from build123d import *

# Parameters (mm, degrees)
F1_DEPTH = 3
F4_R     = 0.5
F6_R     = 0.1
F7_R     = 3
F8_DEPTH = 25
F9_R     = 0.5
F10_R    = 0.2


with BuildPart() as f1:
    # F0 (on Front) → F1 (new body)
    with BuildSketch(Plane.XZ):
        Polygon((1.542941519, -5.5635119126), (5.5896134101, -1.4455294043), (4.0466718911, 4.1179825084), (-1.542941519, 5.5635119126), (-5.5896134101, 1.4455294043), (-4.0466718911, -4.1179825084), align=None)
    extrude(amount=F1_DEPTH)


with BuildPart() as f3:
    # F2 (on Right) → F3 (revolve)
    with BuildSketch(Plane.YZ):
        with BuildLine():
            Line((1.653650824, 0), (1.653650824, 3.2440995908))
            ThreePointArc((1.653650824, 3.2440995908), (0.8126995328, 3.9784778483), (-0.1744808685, 4.5))
            Line((-0.1744808685, 4.5), (-0.1744808685, 0))
            Line((-0.1744808685, 0), (1.653650824, 0))
        make_face()
    revolve(axis=Axis((0, -1.6547753563, 0), (0, -1, 0)))

    # F4
    f4_edges = [f3.edges().sort_by_distance(p)[0] for p in [
        (0, 1.653651, -3.2441),
    ]]
    fillet(f4_edges, radius=F4_R)

    # F5: union F1
    add(f1.part)

    # F6
    f6_edges = [f3.edges().sort_by_distance(p)[0] for p in [
        (0, 0, -4.428349),
    ]]
    fillet(f6_edges, radius=F6_R)

    # F7 (on face) → F8 (cut)
    with BuildSketch(Plane(origin=(0, 1.653650824, 0), x_dir=(-1, 0, 0), z_dir=(0, 1, 0))):
        Circle(F7_R)
    extrude(amount=-F8_DEPTH, mode=Mode.SUBTRACT)

    # F9
    f9_edges = [f3.edges().sort_by_distance(p)[0] for p in [
        (-5.589613, -1.5, 1.445529),
        (-4.046672, -1.5, -4.117983),
        (1.542942, -1.5, -5.563512),
        (-1.542942, -1.5, 5.563512),
        (5.589613, -1.5, -1.445529),
        (4.046672, -1.5, 4.117983),
    ]]
    fillet(f9_edges, radius=F9_R)

    # F10
    f10_edges = [f3.edges().sort_by_distance(p)[0] for p in [
        (1.251865, 0, 4.840747),
        (4.818143, 0, 1.336227),
        (5.514727, 0, -1.426163),
        (3.992457, 0, 4.062812),
        (3.566277, 0, -3.504521),
        (1.52227, 0, -5.488975),
        (-1.251865, 0, -4.840747),
        (-3.992457, 0, -4.062812),
        (-4.818143, 0, -1.336227),
        (-5.514727, 0, 1.426163),
        (-3.566277, 0, 3.504521),
        (-1.52227, 0, 5.488975),
    ]]
    fillet(f10_edges, radius=F10_R)


solid = f3.part
Work out the finished part from the listing and answer in its coordinate system (mm). A direction names the side the tool comes from. Coordinates: 2 decimals unless noted, no trailing zeros. Order: outer loops, then holes, each group sorted by start corner. A loop starts at its lowest first (then second) coordinate and runs counter-clockwise, first axis right, second up. Notation, with made-up numbers: (-1.5, -25) - (13.5, -25) arc R20 cw to (13.5, 14) - close; hole circle Ø7 at (-21, 24). An arc over 180 degrees is marked (long way). Put each result on its own line as item: value. Start each with the question number.
1) Find the intervals of material crossed by line 1 (Z direction, x = 0, y = -1.25); line 2 (Z direction, x = 2, y = 0.5); line 3 (X direction, y = -1.4, z = -2.5), in increasing order. Write a range as from..to.
2) For a pull along Z with two mould halves and no side action, classify faces 1 (the cylindrical face through (3, -1, 0)), 2 (the flat face through (-3, -3, -2)), 3 (the cylindrical face through (-1.202, -0.057, -4.792)) as released by +Z, released by -Z, zero draft, split by the parting line, or undercut.
3) For faces 4 (the flat face through (-4.4, 0, -1.5)), 5 (the flat face through (4.83, -1.58, 1.3)), determine the directions among +Z, -Z, +X, -X, +Y, -Y from which every point of the face is accessible in a straight line to the end or side of a thin tool.
4) Find section A-A (y = -2.7). Give the vertices of the cut face in (x, z), plus the area to 3 significant figures.
5) A flat-ended cylindrical pin translates along its axis: pin 1 (1 mm diameter, centred on y = -0.5, z = -4, fed in from -X). Find the tip coordinate at first contact, or state that the pin passes through.
Results list:
1. line 1: z = -5.16..-3, 3..5.16
1. line 2: z = -3.67..-2.24, 2.24..3.67
1. line 3: x = -4.5..-1.66, 1.66..4.55
2. face 1: undercut
2. face 2: zero draft
2. face 3: released by -Z
3. face 4: +Y
3. face 5: +Z, +X, +Y, -Y
4. outline: (-5.51, 1.17) - (-4.12, -3.84) arc R0.5 ccw to (-3.77, -4.19) - (1.26, -5.49) arc R0.5 ccw to (1.75, -5.36) - (5.39, -1.65) arc R0.5 ccw to (5.51, -1.17) - (4.12, 3.84) arc R0.5 ccw to (3.77, 4.19) - (-1.26, 5.49) arc R0.5 ccw to (-1.75, 5.36) - (-5.39, 1.65) arc R0.5 ccw to start; hole circle Ø6 at (0, 0)
4. area: 58.2 mm^2
5. pin 1: stops at x = -4.22
